```python
from build123d import *

# Parameters (mm, degrees)
SKETCH1_R                   = 70
SKETCH1_R_2                 = 30
SKETCH1_R_3                 = 3
SKETCH1_W                   = 2
SKETCH1_H                   = 5
SKETCH1_W_2                 = 22.5
SKETCH1_H_2                 = 12
SKETCH1_W_3                 = 5
SKETCH1_H_3                 = 2
Y_KSEKLIK_EKSTR_ZYON1_DEPTH = 2
SKETCH3_W                   = 2
SKETCH3_H                   = 2
SKETCH3_W_2                 = 3
BOSS_EXTRUDE1_DEPTH         = 2
SKETCH5_W                   = 5
SKETCH5_H                   = 2
CUT_EXTRUDE1_DEPTH          = 2
SKETCH6_W                   = 2
SKETCH6_H                   = 2
SKETCH6_W_2                 = 3
BOSS_EXTRUDE3_DEPTH         = 2
SKETCH8_W                   = 5
SKETCH8_H                   = 2
CUT_EXTRUDE2_DEPTH          = 2
SKETCH9_W                   = 2
SKETCH9_H                   = 2
SKETCH9_H_2                 = 3
BOSS_EXTRUDE4_DEPTH         = 2
SKETCH10_W                  = 2
SKETCH10_H                  = 2
SKETCH10_H_2                = 3
BOSS_EXTRUDE5_DEPTH         = 2
SKETCH12_W                  = 2
SKETCH12_H                  = 5
CUT_EXTRUDE4_DEPTH          = 2
SKETCH13_W                  = 2
SKETCH13_H                  = 5
CUT_EXTRUDE5_DEPTH          = 2
SKETCH14_W                  = 3
SKETCH14_H                  = 2
SKETCH14_W_2                = 2
BOSS_EXTRUDE6_DEPTH         = 2
SKETCH15_W                  = 5
SKETCH15_H                  = 2
CUT_EXTRUDE6_DEPTH          = 2
SKETCH16_W                  = 3
SKETCH16_H                  = 2
SKETCH16_W_2                = 2
BOSS_EXTRUDE9_DEPTH         = 2
SKETCH17_W                  = 5
SKETCH17_H                  = 2
CUT_EXTRUDE7_DEPTH          = 2
SKETCH18_W                  = 2
SKETCH18_H                  = 3
SKETCH18_H_2                = 2
BOSS_EXTRUDE10_DEPTH        = 2
SKETCH19_W                  = 2
SKETCH19_H                  = 5
CUT_EXTRUDE8_DEPTH          = 2
SKETCH20_W                  = 3
SKETCH20_H                  = 10
SKETCH20_W_2                = 10
SKETCH20_H_2                = 3
SKETCH20_H_3                = 5
CUT_EXTRUDE9_DEPTH          = 2


with BuildPart() as part:
    # Sketch1 → Yükseklik-Ekstrüzyon1 (new body)
    with BuildSketch(Plane(origin=(0, 0, 0), x_dir=(1, 0, 0), z_dir=(0, 1, 0))):
        with Locations(Location((0, 0, 0), (0, 0, 270))):
            Circle(SKETCH1_R)
        with Locations(Location((0, 0, 0), (0, 0, 270))):
            Circle(SKETCH1_R_2, mode=Mode.SUBTRACT)
        with Locations(Location((39.748737342, 0, 0), (0, 0, 270))):
            Circle(SKETCH1_R_3, mode=Mode.SUBTRACT)
        with Locations(Location((-39.748737342, 0, 0), (0, 0, 270))):
            Circle(SKETCH1_R_3, mode=Mode.SUBTRACT)
        with Locations(Location((0, 39.748737342, 0), (0, 0, 270))):
            Circle(SKETCH1_R_3, mode=Mode.SUBTRACT)
        with Locations((-29, 27.5)):
            Rectangle(SKETCH1_W, SKETCH1_H, mode=Mode.SUBTRACT)
        with Locations((29, 27.5)):
            Rectangle(SKETCH1_W, SKETCH1_H, mode=Mode.SUBTRACT)
        with Locations((-29, -27.5)):
            Rectangle(SKETCH1_W, SKETCH1_H, mode=Mode.SUBTRACT)
        with Locations((29, -27.5)):
            Rectangle(SKETCH1_W, SKETCH1_H, mode=Mode.SUBTRACT)
        with Locations((-39.748737342, 39.748737342)):
            Rectangle(SKETCH1_W, SKETCH1_H, mode=Mode.SUBTRACT)
        with Locations((39.748737342, 39.748737342)):
            Rectangle(SKETCH1_W, SKETCH1_H, mode=Mode.SUBTRACT)
        with Locations((39.748737342, -39.748737342)):
            Rectangle(SKETCH1_W, SKETCH1_H, mode=Mode.SUBTRACT)
        with Locations((-39.748737342, -39.748737342)):
            Rectangle(SKETCH1_W, SKETCH1_H, mode=Mode.SUBTRACT)
        with Locations((0, -39.748737342)):
            Rectangle(SKETCH1_W_2, SKETCH1_H_2, mode=Mode.SUBTRACT)
        with Locations((-64.748737342, 4)):
            Rectangle(SKETCH1_W_3, SKETCH1_H_3, mode=Mode.SUBTRACT)
        with Locations((-64.748737342, -4)):
            Rectangle(SKETCH1_W_3, SKETCH1_H_3, mode=Mode.SUBTRACT)
        with Locations((-54.748737342, -4)):
            Rectangle(SKETCH1_W_3, SKETCH1_H_3, mode=Mode.SUBTRACT)
        with Locations((-54.748737342, 4)):
            Rectangle(SKETCH1_W_3, SKETCH1_H_3, mode=Mode.SUBTRACT)
        with Locations((-4, 64.748737342)):
            Rectangle(SKETCH1_W, SKETCH1_H, mode=Mode.SUBTRACT)
        with Locations((-4, 54.748737342)):
            Rectangle(SKETCH1_W, SKETCH1_H, mode=Mode.SUBTRACT)
        with Locations((4, 54.748737342)):
            Rectangle(SKETCH1_W, SKETCH1_H, mode=Mode.SUBTRACT)
        with Locations((4, 64.748737342)):
            Rectangle(SKETCH1_W, SKETCH1_H, mode=Mode.SUBTRACT)
        with Locations((54.748737342, 4)):
            Rectangle(SKETCH1_W_3, SKETCH1_H_3, mode=Mode.SUBTRACT)
        with Locations((54.748737342, -4)):
            Rectangle(SKETCH1_W_3, SKETCH1_H_3, mode=Mode.SUBTRACT)
        with Locations((64.748737342, 4)):
            Rectangle(SKETCH1_W_3, SKETCH1_H_3, mode=Mode.SUBTRACT)
        with Locations((64.748737342, -4)):
            Rectangle(SKETCH1_W_3, SKETCH1_H_3, mode=Mode.SUBTRACT)
        with Locations((-4, -54.748737342)):
            Rectangle(SKETCH1_W, SKETCH1_H, mode=Mode.SUBTRACT)
        with Locations((4, -54.748737342)):
            Rectangle(SKETCH1_W, SKETCH1_H, mode=Mode.SUBTRACT)
        with Locations((4, -64.748737342)):
            Rectangle(SKETCH1_W, SKETCH1_H, mode=Mode.SUBTRACT)
        with Locations((-4, -64.748737342)):
            Rectangle(SKETCH1_W, SKETCH1_H, mode=Mode.SUBTRACT)
    extrude(amount=Y_KSEKLIK_EKSTR_ZYON1_DEPTH)

    # Sketch3 → Boss-Extrude1 (add)
    with BuildSketch(Plane(origin=(0, 2, 0), x_dir=(1, 0, 0), z_dir=(0, 1, 0))):
        with Locations((-66.248737342, 4)):
            Rectangle(SKETCH3_W, SKETCH3_H)
        with Locations((-53.748737342, 4)):
            Rectangle(SKETCH3_W_2, SKETCH3_H)
    extrude(amount=-BOSS_EXTRUDE1_DEPTH)

    # Sketch5 → Cut-Extrude1 (cut)
    with BuildSketch(Plane(origin=(0, 2, 0), x_dir=(1, 0, 0), z_dir=(0, 1, 0))):
        with Locations((-59.748737342, 4)):
            Rectangle(SKETCH5_W, SKETCH5_H)
    extrude(amount=-CUT_EXTRUDE1_DEPTH, mode=Mode.SUBTRACT)

    # Sketch6 → Boss-Extrude3 (add)
    with BuildSketch(Plane(origin=(0, 2, 0), x_dir=(1, 0, 0), z_dir=(0, 1, 0))):
        with Locations((-66.248737342, -4)):
            Rectangle(SKETCH6_W, SKETCH6_H)
        with Locations((-53.748737342, -4)):
            Rectangle(SKETCH6_W_2, SKETCH6_H)
    extrude(amount=-BOSS_EXTRUDE3_DEPTH)

    # Sketch8 → Cut-Extrude2 (cut)
    with BuildSketch(Plane(origin=(0, 2, 0), x_dir=(1, 0, 0), z_dir=(0, 1, 0))):
        with Locations((-59.748737342, -4)):
            Rectangle(SKETCH8_W, SKETCH8_H)
    extrude(amount=-CUT_EXTRUDE2_DEPTH, mode=Mode.SUBTRACT)

    # Sketch9 → Boss-Extrude4 (add)
    with BuildSketch(Plane(origin=(0, 2, 0), x_dir=(1, 0, 0), z_dir=(0, 1, 0))):
        with Locations((4, 66.248737342)):
            Rectangle(SKETCH9_W, SKETCH9_H)
        with Locations((4, 53.748737342)):
            Rectangle(SKETCH9_W, SKETCH9_H_2)
    extrude(amount=-BOSS_EXTRUDE4_DEPTH)

    # Sketch10 → Boss-Extrude5 (add)
    with BuildSketch(Plane(origin=(0, 2, 0), x_dir=(1, 0, 0), z_dir=(0, 1, 0))):
        with Locations((-4, 66.248737342)):
            Rectangle(SKETCH10_W, SKETCH10_H)
        with Locations((-4, 53.748737342)):
            Rectangle(SKETCH10_W, SKETCH10_H_2)
    extrude(amount=-BOSS_EXTRUDE5_DEPTH)

    # Sketch12 → Cut-Extrude4 (cut)
    with BuildSketch(Plane(origin=(0, 2, 0), x_dir=(1, 0, 0), z_dir=(0, 1, 0))):
        with Locations((-4, 59.748737342)):
            Rectangle(SKETCH12_W, SKETCH12_H)
    extrude(amount=-CUT_EXTRUDE4_DEPTH, mode=Mode.SUBTRACT)

    # Sketch13 → Cut-Extrude5 (cut)
    with BuildSketch(Plane(origin=(0, 2, 0), x_dir=(1, 0, 0), z_dir=(0, 1, 0))):
        with Locations((4, 59.748737342)):
            Rectangle(SKETCH13_W, SKETCH13_H)
    extrude(amount=-CUT_EXTRUDE5_DEPTH, mode=Mode.SUBTRACT)

    # Sketch14 → Boss-Extrude6 (add)
    with BuildSketch(Plane(origin=(0, 2, 0), x_dir=(1, 0, 0), z_dir=(0, 1, 0))):
        with Locations((53.748737342, 4)):
            Rectangle(SKETCH14_W, SKETCH14_H)
        with Locations((66.248737342, 4)):
            Rectangle(SKETCH14_W_2, SKETCH14_H)
    extrude(amount=-BOSS_EXTRUDE6_DEPTH)

    # Sketch15 → Cut-Extrude6 (cut)
    with BuildSketch(Plane(origin=(0, 2, 0), x_dir=(1, 0, 0), z_dir=(0, 1, 0))):
        with Locations((59.748737342, 4)):
            Rectangle(SKETCH15_W, SKETCH15_H)
    extrude(amount=-CUT_EXTRUDE6_DEPTH, mode=Mode.SUBTRACT)

    # Sketch16 → Boss-Extrude9 (add)
    with BuildSketch(Plane(origin=(0, 2, 0), x_dir=(1, 0, 0), z_dir=(0, 1, 0))):
        with Locations((53.748737342, -4)):
            Rectangle(SKETCH16_W, SKETCH16_H)
        with Locations((66.248737342, -4)):
            Rectangle(SKETCH16_W_2, SKETCH16_H)
    extrude(amount=-BOSS_EXTRUDE9_DEPTH)

    # Sketch17 → Cut-Extrude7 (cut)
    with BuildSketch(Plane(origin=(0, 2, 0), x_dir=(1, 0, 0), z_dir=(0, 1, 0))):
        with Locations((59.748737342, -4)):
            Rectangle(SKETCH17_W, SKETCH17_H)
    extrude(amount=-CUT_EXTRUDE7_DEPTH, mode=Mode.SUBTRACT)

    # Sketch18 → Boss-Extrude10 (add)
    with BuildSketch(Plane(origin=(0, 2, 0), x_dir=(1, 0, 0), z_dir=(0, 1, 0))):
        with Locations((-4, -53.748737342)):
            Rectangle(SKETCH18_W, SKETCH18_H)
        with Locations((-4, -66.248737342)):
            Rectangle(SKETCH18_W, SKETCH18_H_2)
        with Locations((4, -66.248737342)):
            Rectangle(SKETCH18_W, SKETCH18_H_2)
        with Locations((4, -53.748737342)):
            Rectangle(SKETCH18_W, SKETCH18_H)
    extrude(amount=-BOSS_EXTRUDE10_DEPTH)

    # Sketch19 → Cut-Extrude8 (cut)
    with BuildSketch(Plane(origin=(0, 2, 0), x_dir=(1, 0, 0), z_dir=(0, 1, 0))):
        with Locations((4, -59.748737342)):
            Rectangle(SKETCH19_W, SKETCH19_H)
        with Locations((-4, -59.748737342)):
            Rectangle(SKETCH19_W, SKETCH19_H)
    extrude(amount=-CUT_EXTRUDE8_DEPTH, mode=Mode.SUBTRACT)

    # Sketch20 → Cut-Extrude9 (cut)
    with BuildSketch(Plane(origin=(0, 2, 0), x_dir=(1, 0, 0), z_dir=(0, 1, 0))):
        with Locations((-4, 60.248737342)):
            Rectangle(SKETCH20_W, SKETCH20_H)
        with Locations((4, 60.248737342)):
            Rectangle(SKETCH20_W, SKETCH20_H)
        with Locations((60.248737342, 4)):
            Rectangle(SKETCH20_W_2, SKETCH20_H_2)
        with Locations((60.248737342, -4)):
            Rectangle(SKETCH20_W_2, SKETCH20_H_2)
        with Locations((4, -60.248737342)):
            Rectangle(SKETCH20_W, SKETCH20_H)
        with Locations((-4, -60.248737342)):
            Rectangle(SKETCH20_W, SKETCH20_H)
        with Locations((-60.248737342, 4)):
            Rectangle(SKETCH20_W_2, SKETCH20_H_2)
        with Locations((-60.248737342, -4)):
            Rectangle(SKETCH20_W_2, SKETCH20_H_2)
        with Locations((-29, 27.5)):
            Rectangle(SKETCH20_W, SKETCH20_H_3)
        with Locations((-39.748737342, 39.748737342)):
            Rectangle(SKETCH20_W, SKETCH20_H_3)
        with Locations((29, 27.5)):
            Rectangle(SKETCH20_W, SKETCH20_H_3)
        with Locations((39.748737342, 39.748737342)):
            Rectangle(SKETCH20_W, SKETCH20_H_3)
        with Locations((29, -27.5)):
            Rectangle(SKETCH20_W, SKETCH20_H_3)
        with Locations((39.748737342, -39.748737342)):
            Rectangle(SKETCH20_W, SKETCH20_H_3)
        with Locations((-29, -27.5)):
            Rectangle(SKETCH20_W, SKETCH20_H_3)
        with Locations((-39.748737342, -39.748737342)):
            Rectangle(SKETCH20_W, SKETCH20_H_3)
    extrude(amount=-CUT_EXTRUDE9_DEPTH, mode=Mode.SUBTRACT)


solid = part.part
```
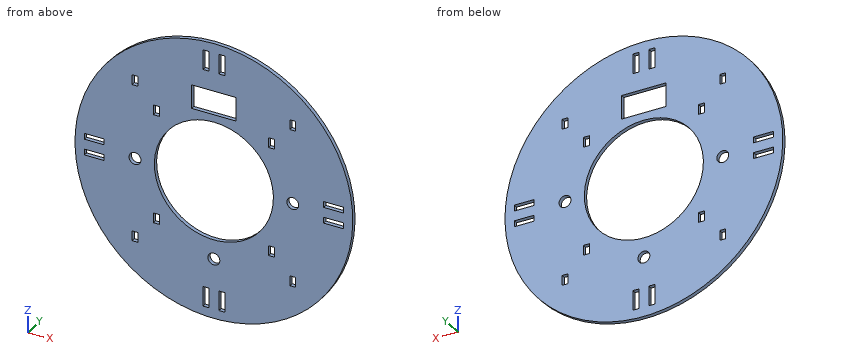
Input: part model. Units: mm. Frame: model coordinates. Round coordinates to 2 decimals unless told otherwise and drop trailing zeros. Loops run counter-clockwise (first coordinate to the right, second up) from the corner with the lowest first, then second, coordinate; pieces in that order, holes last. Notation, with made-up numbers: (7, -11) -> (47, -11) arc R35 cw to (47, 28) -> close; hole circle Ø1 at (20.25, 32.5). An arc over 180 degrees is marked (long way). Write each question's results on one line, items separated by ' | '.
1. First-contact query: P1, Ø0.6, axis at y = 0.5, z = -3.5, coming from the +X side; P2, Ø4, axis at x = -41.5, z = -15, coming from the -Y side; P3, Ø0.6, axis at y = 1, z = -40, coming from the -X side; P4, Ø1, axis at x = -29.5, y = 1, coming from the +Z side. Flat tips, straight axial feed; report the tip coordinate or a pass-through.
Geometry results:
P1: x = 69.93 | P2: y = 0 | P3: x = -57.65 | P4: z = 63.71
2. Section B-B (x = 0). Return loops of the section in (y, z), and give its area (3 significant figures).
Geometry results:
outline: (0, -70) -> (2, -70) -> (2, -42.75) -> (0, -42.75) -> close; (0, -36.75) -> (2, -36.75) -> (2, -30) -> (0, -30) -> close; (0, 30) -> (2, 30) -> (2, 33.75) -> (0, 33.75) -> close; (0, 45.75) -> (2, 45.75) -> (2, 70) -> (0, 70) -> close | area: 124 mm2
3. Ray query, line 1 (X direction, y = 1, z = 0); line 2 (X direction, y = 1, z = -2); line 3 (Z direction, x = -40.5, y = 1.3). Return the intervals inside material, ascending. Write a range as from..to.
Geometry results:
line 1: -70..-42.75, -36.75..-30, 30..36.75, 42.75..70 | line 2: -69.97..-41.98, -37.51..-29.93, 29.93..37.51, 41.98..69.97 | line 3: -57.09..-42.25, -37.25..-2.9, 2.9..37.25, 42.25..57.09
4. Section D-D (z = -21). Return loops of the section in (x, y).
Geometry results:
outline: (-66.78, 0) -> (-21.42, 0) -> (-21.42, 2) -> (-66.78, 2) -> close; (21.42, 0) -> (66.78, 0) -> (66.78, 2) -> (21.42, 2) -> close
5. Section C-C (x = 17.5). Return loops of the section in (y, z), and give its area (3 significant figures).
Geometry results:
outline: (0, -67.78) -> (2, -67.78) -> (2, -24.37) -> (0, -24.37) -> close; (0, 24.37) -> (2, 24.37) -> (2, 67.78) -> (0, 67.78) -> close | area: 174 mm2
6. Section A-A (z = 0). Return loops of the section in (x, y).
Geometry results:
outline: (-70, 0) -> (-42.75, 0) -> (-42.75, 2) -> (-70, 2) -> close; (-36.75, 0) -> (-30, 0) -> (-30, 2) -> (-36.75, 2) -> close; (30, 0) -> (36.75, 0) -> (36.75, 2) -> (30, 2) -> close; (42.75, 0) -> (70, 0) -> (70, 2) -> (42.75, 2) -> close
